Verification items for the finished model (mm, model axes). A direction names the side the tool comes from. Round coordinates to 2 decimals unless told otherwise and drop trailing zeros. Order: outer loops, then holes, each group sorted by start corner. A loop starts at its lowest first (then second) coordinate and runs counter-clockwise, first axis right, second up. Notation, with made-up numbers: M 12.5,47.25 L 24.5,47.25 A28 cw 24.5,66.25 Z; hole C -17.5,51 d8. An arc over 180 degrees is marked long. Use CSV: the item, a comma, the result in double quotes. Start each with the question number.
Q1. Set-up check for faces 4 (the face through (4, 29, -98.28)), 5 (the face through (4, 42, -17)), 6 (the face through (4, 6, -21)), 7 (the face through (4, 21, -10)): record each of +Z, -Z, +X, -X, +Y, -Y from which the full face is reachable in a straight line by a thin tool's end or side.
Q2. Gauge pin test, flat ends, axial feed: pin 1 Ø2.5 at (y, z) = (41.5, -74.28) entering from +X (3 decimals); pin 2 Ø1 at (x, y) = (4, 37) entering from -Z; pin 3 Ø2.5 at (x, z) = (2.5, -19.5) entering from +Y. Record the tip position at first contact, or that the pin passes through.
Q3. Mould release check, pull along X, two halves, no side actions. Record for faces 1 (the face through (8, 32, -53)), 2 (the face through (4, 13, -10)), 3 (the face through (3.94, 45.7, -100.22)): +X half, -X half, draft (parallel to the pull), parting line (faces both ways), or undercut.
Q4. Sectioned sample at A-A (y = 46.5). Enter the section's corners in (x, z), and give its area (3 significant figures).
Q5. Scan lines: line 1 (Y direction, x = 5.25, z = -60.28); line 2 (Y direction, x = 4, z = -105.5); line 3 (X direction, y = 5, z = -105.25). Record each from-to range of solid material in increasing order.
```python
from build123d import *

# Parameters (mm, degrees)
SKETCH_1_R          = 1.6
SKETCH_1_R_2        = 11.25
SKETCH_1_R_3        = 2.1
EXTRUDE_1_DEPTH     = 8
SKETCH_2_R          = 1.65
CUT_EXTRUDE_1_DEPTH = 10
SKETCH_3_W          = 18
SKETCH_3_H          = 30
SKETCH_3_W_2        = 40
SKETCH_3_H_2        = 16
SKETCH_3_W_3        = 10.28
CUT_EXTRUDE_2_DEPTH = 10
FILLET_1_R          = 4
FILLET_2_R          = 2


with BuildPart() as part:
    # 草图1 → 凸台-拉伸1 (new body)
    with BuildSketch(Plane(origin=(0, 0, 0), x_dir=(0, 0, -1), z_dir=(1, 0, 0))):
        Polygon((0, 42), (0, 0), (108.28, 0), (108.28, 63.5), (45.28, 63.5), (32.866969212, 42), align=None)
        with Locations((46.28, 41.5)):
            Circle(SKETCH_1_R, mode=Mode.SUBTRACT)
        with Locations((60.28, 41.5)):
            Circle(SKETCH_1_R_2, mode=Mode.SUBTRACT)
        with Locations((74.28, 41.5)):
            Circle(SKETCH_1_R, mode=Mode.SUBTRACT)
        with Locations((52.28, 27.643593539)):
            Circle(SKETCH_1_R_3, mode=Mode.SUBTRACT)
        with Locations((60.28, 27.5)):
            Circle(SKETCH_1_R, mode=Mode.SUBTRACT)
        with Locations((68.28, 27.643593539)):
            Circle(SKETCH_1_R_3, mode=Mode.SUBTRACT)
        with Locations((98.28, 46.5)):
            Circle(SKETCH_1_R_3, mode=Mode.SUBTRACT)
        with Locations((60.28, 55.5)):
            Circle(SKETCH_1_R, mode=Mode.SUBTRACT)
        with Locations((68.28, 55.356406461)):
            Circle(SKETCH_1_R_3, mode=Mode.SUBTRACT)
        with Locations((98.28, 58.5)):
            Circle(SKETCH_1_R, mode=Mode.SUBTRACT)
        with Locations((52.28, 55.356406461)):
            Circle(SKETCH_1_R_3, mode=Mode.SUBTRACT)
    extrude(amount=EXTRUDE_1_DEPTH)

    # 草图2 → 切除-拉伸1 (cut)
    with BuildSketch(Plane.XY):
        with Locations((4, 21)):
            Circle(SKETCH_2_R)
        with Locations((4, 29)):
            Circle(SKETCH_2_R)
        with Locations((4, 37)):
            Circle(SKETCH_2_R)
        with Locations(Location((4, 5, 0), (0, 0, 180))):
            Circle(SKETCH_2_R)
        with Locations(Location((4, 13, 0), (0, 0, 180))):
            Circle(SKETCH_2_R)
    cut_extrude_1 = extrude(amount=-CUT_EXTRUDE_1_DEPTH, mode=Mode.SUBTRACT)

    # 镜向1: 切除-拉伸1 across plane
    add(cut_extrude_1.mirror(Plane.XY.offset(-54.14)), mode=Mode.SUBTRACT)

    # 草图3 → 切除-拉伸2 (cut)
    with BuildSketch(Plane(origin=(8, 0, 0), x_dir=(0, 0, -1), z_dir=(1, 0, 0))):
        with Locations((21, 21)):
            Rectangle(SKETCH_3_W, SKETCH_3_H)
        with Locations((58, 14)):
            Rectangle(SKETCH_3_W_2, SKETCH_3_H_2)
        with Locations((91.14, 21)):
            Rectangle(SKETCH_3_W_3, SKETCH_3_H)
    extrude(amount=-CUT_EXTRUDE_2_DEPTH, mode=Mode.SUBTRACT)

    # 圆角1
    fillet_1_edges = [part.edges().sort_by_distance(p)[0] for p in [
        (4, 6, -12),
        (4, 36, -12),
        (4, 36, -30),
        (4, 6, -30),
        (4, 6, -38),
        (4, 22, -38),
        (4, 22, -78),
        (4, 6, -78),
        (4, 6, -86),
        (4, 36, -86),
        (4, 36, -96.28),
        (4, 6, -96.28),
    ]]
    fillet(fillet_1_edges, radius=FILLET_1_R)

    # 圆角2
    fillet_2_edges = [part.edges().sort_by_distance(p)[0] for p in [
        (4, 0, -108.28),
        (4, 0, 0),
        (4, 42, 0),
        (4, 42, -32.866969212),
        (4, 63.5, -45.28),
        (4, 63.5, -108.28),
    ]]
    fillet(fillet_2_edges, radius=FILLET_2_R)


solid = part.part
```
Verdict:
1,face 4,"-Z"
1,face 5,"+Z, +X, -X, +Y"
1,face 6,"+X, -X"
1,face 7,"+Z"
2,pin 1,"passes through"
2,pin 2,"stops at z = -98.28"
2,pin 3,"stops at y = 42"
3,face 1,"+X half"
3,face 2,"undercut"
3,face 3,"draft"
4,outline,"M 0,-108.28 L 8,-108.28 L 8,-100.38 L 0,-100.38 Z; M 0,-96.18 L 8,-96.18 L 8,-70.36 L 0,-70.36 Z; M 0,-50.2 L 8,-50.2 L 8,-35.47 L 0,-35.47 Z"
4,area,"388 mm²"
5,line 1,"y = 0 to 6, 22 to 25.9, 29.1 to 30.25, 52.75 to 53.9, 57.1 to 63.5"
5,line 2,"y = 0 to 3.35, 6.65 to 11.35, 14.65 to 19.35, 22.65 to 27.35, 30.65 to 35.35, 38.65 to 63.5"
5,line 3,"x = 0 to 2.35, 5.65 to 8"
